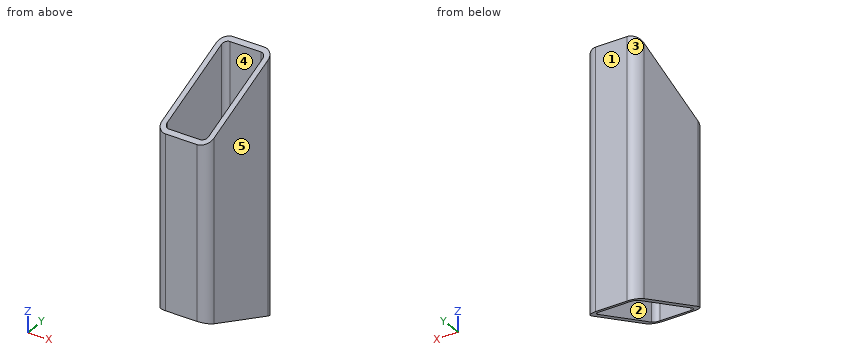
Autodesk Inventor part; units mm, degrees
ref_plane "Start Plane" through (0, 0, 0) normal (0, 0, 1) x (1, 0, 0)
ref_plane "End Plane" through (0, 0, 100) normal (0, 0, 1) x (1, 0, 0)
ref_plane "Work Plane4" through (0, 20, 100) normal (0, -0.3827, 0.9239) x (1, 0, 0)
ref_plane "Start Plane" through (0, 0, 0) normal (0, 0, 1) x (1, 0, 0)
ref_plane "End Plane" through (0, 0, 100) normal (0, 0, 1) x (1, 0, 0)
sketch "Sketch" plane through (0, 0, 0) normal (0, 0, 1) x (1, 0, 0)
  line L0 (-10, -16) -> (-10, 16)
  line L1 (-6, 20) -> (6, 20)
  line L2 (10, 16) -> (10, -16)
  line L3 (6, -20) -> (-6, -20)
  arc A0 (-10, -16) -> (-6, -20) centre (-6, -16) ccw
  arc A1 (10, 16) -> (6, 20) centre (6, 16) ccw
  arc A2 (-6, 20) -> (-10, 16) centre (-6, 16) ccw
  arc A3 (6, -20) -> (10, -16) centre (6, -16) ccw
  arc A4 (-6, 18) -> (-8, 16) centre (-6, 16) ccw
  line L4 (-6, 18) -> (6, 18)
  arc A5 (8, 16) -> (6, 18) centre (6, 16) ccw
  line L5 (8, 16) -> (8, -16)
  arc A6 (6, -18) -> (8, -16) centre (6, -16) ccw
  line L6 (6, -18) -> (-6, -18)
  arc A7 (-8, -16) -> (-6, -18) centre (-6, -16) ccw
  line L7 (-8, -16) -> (-8, 16)
  line L8 (0, 29.1598) -> (0, -29.1598) construction
  line L9 (-15.1598, 0) -> (15.1598, 0) construction
  dimension "d7" = 4
  dimension "d9" = 20
  dimension "d11" = 40
  dimension "d12" = 2
  dimension "d15" = 10
  dimension "d16" = 20
extrude "Body" add sketch "Sketch" along normal up to surface (100 mm away) from surface at 0
sketch "Sketch3" plane through (0, 0, 0) normal (0, 0, 1) x (1, 0, 0)
  line L0 (0, 0) -> (10, 0)
ref_plane "Work Plane3" through (0, 0, 0) normal (0, -1, 0) x (1, 0, 0)
ref_plane "Work Plane4" through (0, 20, 100) normal (0, -0.3827, 0.9239) x (1, 0, 0)
split "Split1" plane through (0, 20, 100) removes the side toward (0, -0.3827, 0.9239)
ref_plane "Work Plane5" through (0, 20, 0) normal (0, -0.3827, -0.9239) x (1, 0, 0)
split "Split2" plane through (0, 20, 0) removes the side toward (0, -0.3827, -0.9239)
sketch "Sketch4" plane through (0, 0, 0) normal (0, -1, 0) x (1, 0, 0)
  line L0 (-2, 0) -> (12, 0)
  line L1 (-2, 100) -> (12, 100)
  dimension "d18" = 100
equation "\"d7\" = G_IR"
equation "\"d9\" = G_W"
equation "\"d11\" = G_H"
equation "\"d12\" = G_T"
equation "\"d15\" = 0.5 * d9"
equation "\"d16\" = 0.5 * d11"
equation "\"d3\" = G_L"
equation "\"G_W\" = 20"
equation "\"G_H\" = 40"
equation "\"G_T\" = 2"
equation "\"G_IR\" = 4"
equation "\"G_L\" = d18"
equation "\"G_OFFSET_START\" = 0"
equation "\"G_OFFSET_END\" = 0"
properties part number "ISO 4019 - 40x20x2 - 100" material "Steel, Mild"
Source: CAD feature listing. Evaluate the final solid. Frame: model axes, mm. Face numbers are marked on the shaded views. A direction names the side the tool comes from. Round coordinates to 2 decimals unless told otherwise and drop trailing zeros. Order: outer loops, then holes, each group sorted by start corner. A loop starts at its lowest first (then second) coordinate and runs counter-clockwise, first axis right, second up. Notation, with made-up numbers: (53, 82) -> (81, 82) arc R27 cw to (81, 108) -> close; hole circle Ø7 at (-11, -10.75). An arc over 180 degrees is marked (long way). One line per item, written item: value. Start each with the question number.
Q1. Access query for the marked faces 1 and 2. Directions: +Z, -Z, +X, -X, +Y, -Y. A direction counts if a zero-diameter tool reaches every point of the face in a straight line with its end or side. Return the directions, or none.
Q2. Material intervals for probe 1 along Y at (x, z) = (-4.5, 44.5); probe 2 along X at (y, z) = (11, 89); probe 3 along Y at (x, z) = (-7.25, 30), sorted ascending.
Q3. Section query B-B (z = 36). Return the cut outline in (x, y).
Q4. Section query C-C (y = 6). Return the cut outline in (x, z), plus the area to 3 significant figures.
Q5. Section query D-D (z = 87.5). Return the cut outline in (x, y), plus the area to 3 significant figures.
Q6. Pin query (flat end, axial travel): pin 1 (4 mm diameter, centred on x = 6.5, y = -6.5, fed in from -Z); pin 2 (3 mm diameter, centred on x = 8, y = 10.5, fed in from -Z); pin 3 (12 mm diameter, centred on x = -3, y = 0, fed in from +Z). Return the tip coordinate at first contact, or that it passes through.
Q7. Draft query along Y for the marked faces 3, 4 and 5. Return one class per face: pulls with the +Y half, pulls with the -Y half, needs draft (parallel to the pull), parting line crosses it, or undercut.
Q8. Section query A-A (x = -2.5). Return the cut outline in (y, z).
Findings below:
1. face 1: +Z, -Z, +X, -X, +Y
1. face 2: +Z, -Z
2. probe 1: -20 to -18, 18 to 20
2. probe 2: -10 to -8, 8 to 10
2. probe 3: -19.8 to -17.56, 17.56 to 19.8
3. outline: (-10, -16) arc R4 ccw to (-6, -20) -> (6, -20) arc R4 ccw to (10, -16) -> (10, 16) arc R4 ccw to (6, 20) -> (-6, 20) arc R4 ccw to (-10, 16) -> close; hole (-8, -16) arc R2 ccw to (-6, -18) -> (6, -18) arc R2 ccw to (8, -16) -> (8, 16) arc R2 ccw to (6, 18) -> (-6, 18) arc R2 ccw to (-8, 16) -> close
4. outline: (-10, 5.8) -> (-8, 5.8) -> (-8, 94.2) -> (-10, 94.2) -> close; (8, 5.8) -> (10, 5.8) -> (10, 94.2) -> (8, 94.2) -> close
4. area: 354 mm²
5. outline: (-10, -10.18) -> (-8, -10.18) -> (-8, 16) arc R2 cw to (-6, 18) -> (6, 18) arc R2 cw to (8, 16) -> (8, -10.18) -> (10, -10.18) -> (10, 16) arc R4 ccw to (6, 20) -> (-6, 20) arc R4 ccw to (-10, 16) -> close
5. area: 148 mm²
6. pin 1: z = 10.43
6. pin 2: z = 3.31
6. pin 3: z = 93.09
7. face 3: pulls with the +Y half
7. face 4: undercut
7. face 5: needs draft
8. outline: (-20, 16.57) -> (-18, 15.74) -> (-18, 84.26) -> (-20, 83.43) -> close; (18, 0.83) -> (20, 0) -> (20, 100) -> (18, 99.17) -> close
